Autodesk Inventor part; units mm, degrees
ref_plane "YZ Plane" through (0, 0, 0) normal (1, 0, 0) x (0, 1, 0)
ref_plane "XZ Plane" through (0, 0, 0) normal (0, 1, 0) x (-1, 0, 0)
ref_plane "XY Plane" through (0, 0, 0) normal (0, 0, 1) x (1, 0, 0)
sketch "Sketch1" plane through (0, 0, 0) normal (0, 0, 1) x (1, 0, 0)
  line L0 (0, 0) -> (220, 0)
  line L1 (220, 0) -> (220, 480)
  line L2 (220, 480) -> (0, 480)
  line L3 (0, 480) -> (0, 0)
  dimension "d0" = 480
  dimension "d1" = 220
extrude "Extrusion1" add sketch "Sketch1" along normal blind 360
sketch "Sketch2" plane through (0, 480, 0) normal (0, 1, 0) x (1, 0, 0)
  line L0 (220, 0) -> (220, -360)
  line L1 (0, 0) -> (220, 0)
  line L2 (220, 0) -> (220, -160)
  line L3 (220, -160) -> (0, -160)
  line L4 (0, -160) -> (0, 0)
  line L5 (20, -20) -> (200, -20)
  line L6 (200, -20) -> (200, -140)
  line L7 (200, -140) -> (20, -140)
  line L8 (20, -140) -> (20, -20)
  line L9 (0, -360) -> (220, -360)
  line L10 (0, -160) -> (220, -160)
  line L11 (220, -160) -> (220, -360)
  line L12 (220, -360) -> (0, -360)
  line L13 (0, -360) -> (0, -160)
  dimension "d4" = 160
  dimension "d5" = 20
  dimension "d6" = 20
  dimension "d7" = 20
  dimension "d8" = 20
extrude "Extrusion2" cut sketch "Sketch2" against normal blind 220 contours L0 L9 L13 L3
sketch "Sketch3" plane through (220, 0, 0) normal (1, 0, 0) x (0, 0, -1)
  line L0 (-20, 240) -> (-20, 20)
  line L1 (-20, 20) -> (-340, 20)
  line L2 (-340, 20) -> (-340, 240)
  line L3 (-160, 260) -> (-360, 260)
  line L4 (-360, 0) -> (-360, 260)
  line L5 (0, 0) -> (-360, 0)
  line L6 (0, 0) -> (0, 480)
  line L7 (-340, 240) -> (-140, 240)
  line L8 (-140, 240) -> (-140, 460)
  line L9 (-140, 460) -> (-20, 460)
  line L10 (-20, 460) -> (-20, 240)
  line L11 (-160, 480) -> (-160, 260)
  line L12 (0, 480) -> (-160, 480)
  dimension "d12" = 20
  dimension "d13" = 20
  dimension "d14" = 20
  dimension "d16" = 20
  dimension "d17" = 20
  dimension "d18" = 20
extrude "Extrusion3" cut sketch "Sketch3" against normal blind 220 contours L0 L1 L2 L7 L8 L9 L10
sketch "Sketch4" plane through (0, 0, 360) normal (0, 0, 1) x (1, 0, 0)
  line L0 (20, 240) -> (200, 240)
  line L1 (200, 240) -> (200, 20)
  line L2 (200, 20) -> (20, 20)
  line L3 (20, 20) -> (20, 240)
  line L4 (220, 260) -> (0, 260)
  line L5 (0, 260) -> (0, 0)
  line L6 (0, 0) -> (220, 0)
  line L7 (220, 0) -> (220, 260)
  dimension "d21" = 20
  dimension "d22" = 20
  dimension "d23" = 20
  dimension "d24" = 20
extrude "Extrusion4" cut sketch "Sketch4" against normal blind 600 contours L0 L1 L2 L3
sketch "Sketch5" plane through (0, 0, 0) normal (0, -1, 0) x (1, 0, 0)
  line L0 (200, 20) -> (200, 0)
  line L1 (20, 340) -> (200, 340)
  line L2 (200, 340) -> (200, 20)
  line L3 (200, 20) -> (20, 20)
  line L4 (20, 20) -> (20, 340)
  point P0 (0, 0)
extrude "Extrusion5" cut sketch "Sketch5" against normal blind 900
sketch "Sketch6" plane through (0, 0, 0) normal (0, 0, -1) x (-1, 0, 0)
  line L0 (-220, 240) -> (-200, 240)
  line L1 (-20, 460) -> (-20, 240)
  line L2 (-200, 240) -> (-20, 240)
  line L3 (-20, 240) -> (-20, 460)
  line L4 (-20, 460) -> (-200, 460)
  line L5 (-200, 460) -> (-200, 240)
  point P0 (0, 0)
extrude "Extrusion6" cut sketch "Sketch6" against normal blind 80
sketch "Sketch7" plane through (20, 260, 160) normal (1, 0, 0) x (0, 0, -1)
  line L0 (20, 200) -> (20, -20)
  line L1 (20, -20) -> (0, -20)
  line L2 (0, -20) -> (0, 0)
  line L3 (0, 0) -> (20, 0)
  line L4 (20, 0) -> (20, -20)
  point P0 (160, -260)
extrude "Extrusion7" add sketch "Sketch7" along normal blind 180
sketch "Sketch8" plane through (0, 0, 0) normal (0, -1, 0) x (1, 0, 0)
  point P0 (0, 0)
sketch "Sketch9" plane through (220, 0, 0) normal (1, 0, 0) x (0, 0, -1)
  line L0 (-360, 0) -> (-360, 260)
  line L1 (-360, 0) -> (-360, 260)
  line L2 (-360, 260) -> (-160, 260)
  line L3 (-160, 480) -> (-20, 480)
  line L4 (-160, 260) -> (-160, 480)
  line L5 (-160, 480) -> (0, 480)
  line L6 (0, 480) -> (0, 0)
  line L7 (0, 0) -> (-360, 0)
extrude "Extrusion8" add sketch "Sketch9" along normal blind 72
sketch "Sketch10" plane through (292, 0, 0) normal (1, 0, 0) x (0, 0, -1)
  line L0 (-340, 20) -> (-340, 240)
  line L1 (-340, 240) -> (-340, 20)
  line L2 (-20, 20) -> (-340, 20)
  line L3 (-340, 20) -> (-20, 20)
  line L4 (0, 460) -> (-20, 460)
  line L5 (-20, 20) -> (-20, 460)
  line L6 (-20, 460) -> (-140, 460)
  line L7 (-140, 240) -> (-340, 240)
  line L8 (-140, 460) -> (-140, 240)
  line L9 (-140, 240) -> (-340, 240)
  point P0 (0, 0)
extrude "Extrusion9" cut sketch "Sketch10" against normal blind 150
sketch "Sketch11" plane through (0, 0, 360) normal (0, 0, 1) x (1, 0, 0)
  line L0 (20, 240) -> (200, 240)
  line L1 (292, 20) -> (200, 20)
  line L2 (200, 240) -> (272, 240)
  line L3 (272, 240) -> (272, 20)
  line L4 (272, 20) -> (200, 20)
  line L5 (200, 20) -> (200, 240)
  line L6 (292, 260) -> (292, 0)
  point P0 (0, 0)
  dimension "d37" = 20
extrude "Extrusion10" cut sketch "Sketch11" against normal blind 900
sketch "Sketch12" plane through (0, 260, 0) normal (0, 1, 0) x (1, 0, 0)
  line L0 (200, -340) -> (200, -160)
  line L1 (200, -160) -> (272, -160)
  line L2 (272, -160) -> (272, -340)
  line L3 (272, -340) -> (200, -340)
  line L4 (200, -340) -> (200, -160)
  line L5 (292, -160) -> (292, -360)
  point P0 (0, 0)
  dimension "d40" = 20
extrude "Extrusion11" cut sketch "Sketch12" against normal blind 900
sketch "Sketch13" plane through (20, 260, 160) normal (0, 0, 1) x (1, 0, 0)
  line L0 (180, 200) -> (0, 200)
  line L1 (252, 0) -> (272, 0)
  line L2 (180, 200) -> (252, 200)
  line L3 (252, 200) -> (252, 0)
  line L4 (252, 0) -> (180, 0)
  line L5 (180, 0) -> (180, 200)
  point P0 (-20, -260)
extrude "Extrusion12" cut sketch "Sketch13" against normal blind 900
sketch "Sketch14" plane through (0, 480, 160) normal (0, 1, 0) x (1, 0, 0)
  line L0 (200, 140) -> (200, 0)
  line L1 (292, 140) -> (272, 140)
  line L2 (200, 0) -> (272, 0)
  line L3 (272, 0) -> (272, 140)
  line L4 (272, 140) -> (200, 140)
  line L5 (200, 140) -> (200, 0)
  point P0 (0, 160)
extrude "Extrusion13" cut sketch "Sketch14" against normal blind 900
sketch "Sketch15" plane through (200, 240, 140) normal (1, 0, 0) x (0, 0, -1)
  line L0 (-220, 20) -> (-20, 20)
  line L1 (0, 0) -> (-200, 0)
  line L2 (-20, 20) -> (0, 20)
  line L3 (0, 20) -> (0, 0)
  line L4 (0, 0) -> (-20, 0)
  line L5 (-20, 0) -> (-20, 20)
  point P0 (140, -240)
extrude "Extrusion14" add sketch "Sketch15" along normal up to next
sketch "Sketch16" plane through (200, 240, 0) normal (-1, 0, 0) x (0, 0, 1)
  line L0 (20, 20) -> (0, 20)
  line L1 (20, 0) -> (20, -220)
  line L2 (0, 20) -> (20, 20)
  line L3 (20, 20) -> (20, 0)
  line L4 (20, 0) -> (0, 0)
  line L5 (0, 0) -> (0, 20)
  point P0 (0, -240)
extrude "Extrusion15" cut sketch "Sketch16" against normal up to surface (72 mm away) from surface at 0
sketch "Sketch17" plane through (0, 0, 0) normal (0, -1, 0) x (1, 0, 0)
  line L0 (292, 360) -> (0, 360)
  line L1 (292, 360) -> (292, 0)
  line L2 (0, 360) -> (292, 360)
  line L3 (292, 360) -> (292, 0)
  line L4 (292, 0) -> (0, 0)
  line L5 (0, 0) -> (0, 360)
  point P0 (0, 0)
extrude "Extrusion16" cut sketch "Sketch17" against normal blind 20
sketch "Sketch18" plane through (0, 0, 360) normal (0, 0, 1) x (1, 0, 0)
  line L0 (0, 20) -> (292, 20)
  line L1 (292, 20) -> (292, 40)
  line L2 (292, 40) -> (0, 40)
  line L3 (0, 40) -> (0, 20)
  point P0 (0, 0)
  dimension "d53" = 20
extrude "Extrusion17" add sketch "Sketch18" against normal blind 360
sketch "Sketch19" plane through (0, 20, 0) normal (0, -1, 0) x (1, 0, 0)
  line L0 (20, 360) -> (20, 340)
  line L1 (20, 340) -> (272, 340)
  line L2 (272, 340) -> (272, 20)
  line L3 (272, 20) -> (20, 20)
  line L4 (20, 20) -> (20, 340)
  point P0 (0, 0)
extrude "Extrusion18" cut sketch "Sketch19" against normal blind 60
properties part number "fuel tank housing"
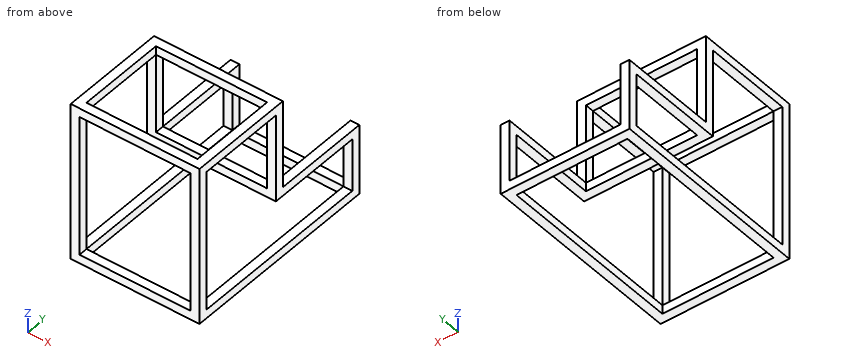
Can you work these out from the model? Positions are in its coordinate system, mm. Give positions to 0.01 mm unless a question says otherwise; leave off trailing zeros. Order: outer loops, then holes, each group sorted by start corner. A loop starts at its lowest first (then second) coordinate and runs counter-clockwise, first axis right, second up. Notation, with made-up numbers: M 63.25,10 L 114.25,10 A8 ccw 114.25,23 Z; hole C 61,15 d9. An arc over 180 degrees is marked long. Write item = value, one per line. Start each with the question number.
Q1. Suppose I cut it at B-B (y = 177). Write out the boundary of the cut face in (x, z).
Q2. I need wall thicknesses on probe 1 along Z at (x, y) = (140, 253.5); probe 2 along Z at (x, y) = (12, 448); probe 3 along X at (y, z) = (391, 158.5). Which ranges of each line are inside material? Lowest first, please. Write a range as [from, to].
Q3. Suppose I cut it at C-C (x = 69). Write out the boundary of the cut face in (y, z).
Q4. Suppose I cut it at A-A (z = 301). Write out the boundary of the cut face in (x, y), plus the area to 3 significant figures.
Q5. Will these pins go through, and if not, where does the flat tip stop? pin 1 Ø16 at (x, y) = (286.5, 408) entering from +Z; pin 2 Ø22 at (x, z) = (12.5, 230) entering from +Y; pin 3 Ø6 at (x, y) = (174.5, 467) entering from +Z.
Check result:
q1.outline = M 0,0 L 20,0 L 20,20 L 0,20 Z; M 0,340 L 20,340 L 20,360 L 0,360 Z; M 272,0 L 292,0 L 292,20 L 272,20 Z; M 272,340 L 292,340 L 292,360 L 272,360 Z
q2.probe_1 = [140, 160], [340, 360]
q2.probe_2 = [0, 20], [140, 160]
q2.probe_3 = [0, 20], [272, 292]
q3.outline = M 20,0 L 40,0 L 40,20 L 20,20 Z; M 20,340 L 40,340 L 40,360 L 20,360 Z; M 240,140 L 260,140 L 260,160 L 240,160 Z; M 240,340 L 260,340 L 260,360 L 240,360 Z; M 460,0 L 480,0 L 480,20 L 460,20 Z
q4.outline = M 0,20 L 20,20 L 20,40 L 0,40 Z; M 0,240 L 20,240 L 20,260 L 0,260 Z; M 272,20 L 292,20 L 292,40 L 272,40 Z; M 272,240 L 292,240 L 292,260 L 272,260 Z
q4.area = 1,600 mm2
q5.pin_1 = 160
q5.pin_2 = 260
q5.pin_3 = 20
